Study the drawing (mm; zero at the part's minimum x, y, z) and answer. A direction names the side the tool comes from. Coordinates: 2 decimals unless noted, no trailing zeros. Order: outer loops, then holes, each group sorted by start corner. A loop starts at its lowest first (then second) coordinate and runs counter-clockwise, first axis right, second up.
1. The part is cut by section D-D, the plane z = 16.75. Give the vertices of the cut face in (x, y), then the cut area to 3 significant figures.
2. The part is cut by section B-B, the plane x = 21. Give the vertices of the cut face in (y, z), then the cut area to 3 significant figures.
3. Flat-ended cylindrical pins translate along their axes: pin 1 Ø8 at (x, z) = (14.5, 6) entering from +Y; pin 2 Ø12 at (x, z) = (30.5, 16.5) entering from +Y; pin 3 Ø4.5 at (x, y) = (30, 28) entering from +Z; pin 4 Ø6 at (x, z) = (39, 13) entering from +Y. Find the tip coordinate at first contact, or state that the pin passes through.
4. The part is cut by section A-A, the plane y = 6. Give the vertices of the cut face in (x, z).
5. Determine the mould class of the marked faces 1, 2 and 3 for opening direction X: +X half, -X half, draft (parallel to the pull), parting line (faces both ways), or undercut.
6. A tool of negligible diameter and unlimited length cuts with its end or side. For the marked faces 4, 5 and 6, from which of +Z, -Z, +X, -X, +Y, -Y can it reach the whole face along a straight path? Write none if from no direction.
7. The part is cut by section C-C, the plane y = 24.5. Give the vertices of the cut face in (x, z).
8. Find the intervals of material crossed by probe 1 along X at (y, z) = (6.5, 13); probe 2 along Z at (x, y) = (39, 6); probe 3 along Y at (x, z) = (21.5, 18), in increasing order.
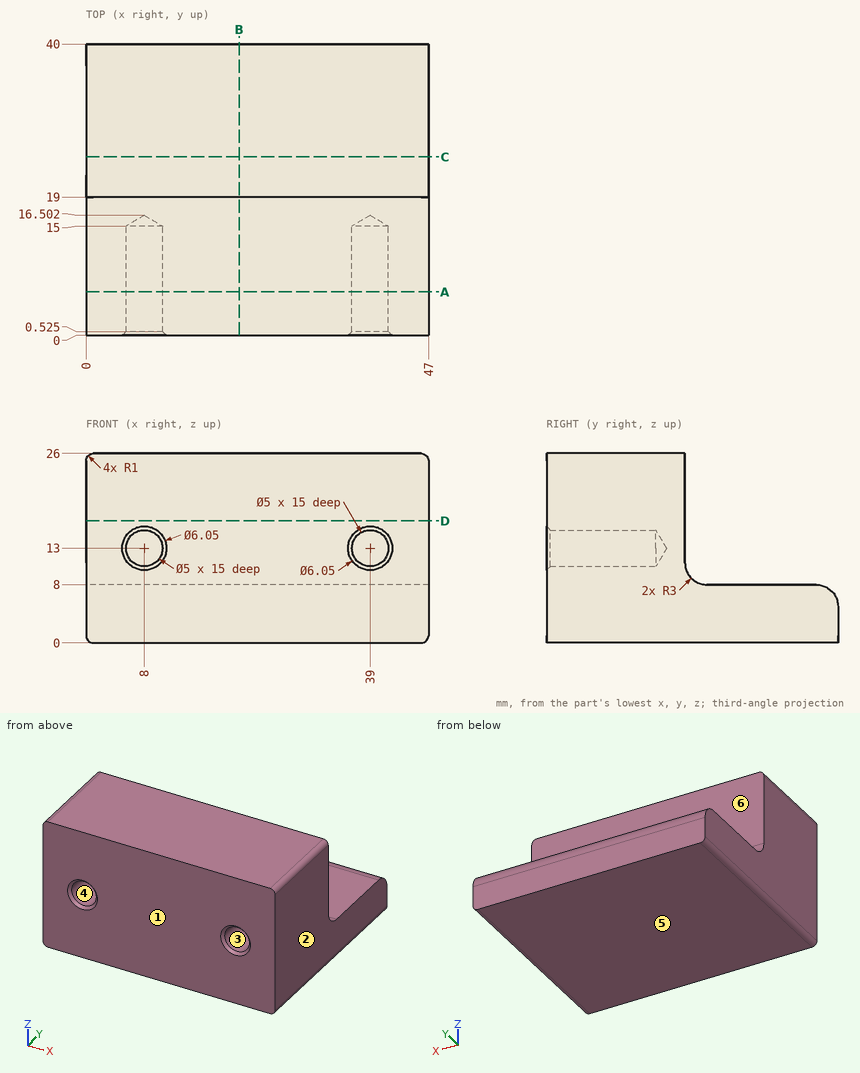
Geometry says:
1. outline: (0, 0) - (47, 0) - (47, 19) - (0, 19) - close
1. area: 893 mm2
2. outline: (0, 0) - (40, 0) - (40, 5) arc R3 ccw to (37, 8) - (22, 8) arc R3 cw to (19, 11) - (19, 26) - (0, 26) - close
2. area: 662 mm2
3. pin 1: stops at y = 40
3. pin 2: stops at y = 19.04
3. pin 3: stops at z = 8
3. pin 4: stops at y = 19.17
4. outline: (0, 1) arc R1 ccw to (1, 0) - (46, 0) arc R1 ccw to (47, 1) - (47, 25) arc R1 ccw to (46, 26) - (1, 26) arc R1 ccw to (0, 25) - close; hole circle Ø5 at (8, 13); hole circle Ø5 at (39, 13)
5. face 1: draft
5. face 2: +X half
5. face 3: undercut
6. face 4: -Y
6. face 5: -Z, +X, -X, +Y, -Y
6. face 6: +Z, +X, -X, +Y
7. outline: (0, 1) arc R1 ccw to (1, 0) - (46, 0) arc R1 ccw to (47, 1) - (47, 8) - (0, 8) - close
8. probe 1: x = 0 to 5.5, 10.5 to 36.5, 41.5 to 47
8. probe 2: z = 0 to 10.5, 15.5 to 26
8. probe 3: y = 0 to 19
